```python
from build123d import *

# Parameters (mm, degrees)
BOSS_EXTRUDE1_DEPTH = 88.9
FILLET2_R           = 0.254
FILLET1_R           = 1.27
SKETCH5_W           = 7.112
SKETCH5_H           = 2.54
BOSS_EXTRUDE2_DEPTH = 177.8


with BuildPart() as part:
    # Sketch3 → Boss-Extrude1 (new body, symmetric)
    with BuildSketch(Plane.XY):
        with BuildLine():
            Line((-12.7, 12.7), (-1.796051224, 1.796051224))
            ThreePointArc((-1.796051224, 1.796051224), (-0.972015918, 2.346654013), (0, 2.54))
            Line((0, 2.54), (0, 4.826))
            Line((0, 4.826), (-1.977846327, 4.826))
            ThreePointArc((-1.977846327, 4.826), (-2.949862246, 5.019345987), (-3.773897552, 5.569948776))
            Line((-3.773897552, 5.569948776), (-7.772528286, 9.56857951))
            ThreePointArc((-7.772528286, 9.56857951), (-7.847628361, 9.946133082), (-7.527553898, 10.16))
            Line((-7.527553898, 10.16), (-3.302, 10.16))
            Line((-3.302, 10.16), (-3.302, 12.7))
            Line((-3.302, 12.7), (-12.7, 12.7))
        make_face()
    extrude(amount=BOSS_EXTRUDE1_DEPTH, both=True)

    # Fillet2
    fillet2_edges = [part.edges().sort_by_distance(p)[0] for p in [
        (-3.302, 12.7, 0),
        (-3.302, 10.16, 0),
    ]]
    fillet(fillet2_edges, radius=FILLET2_R)

    # Mirror1: part across plane


with BuildPart() as part_1:
    add(part.part)
    add(part.part.mirror(Plane(origin=(0, 0, 88.9), x_dir=(0, 0, 1), z_dir=(0.707106781, 0.707106781, 0))))

    # Fillet1
    fillet1_edges = [part_1.edges().sort_by_distance(p)[0] for p in [
        (-12.7, 12.7, 0),
    ]]
    fillet(fillet1_edges, radius=FILLET1_R)

    # Mirror2: part across plane


with BuildPart() as part_2:
    add(part_1.part)
    add(part_1.part.mirror(Plane(origin=(0, 0, 88.9), x_dir=(0, 0, 1), z_dir=(0, 1, 0))))

    # Mirror5: part across plane


with BuildPart() as part_3:
    add(part_2.part)
    add(part_2.part.mirror(Plane(origin=(0, 0, 88.9), x_dir=(0, 0, 1), z_dir=(-1, 0, 0))))

    # Sketch5 → Boss-Extrude2 (add, through all)
    with BuildSketch(Plane.XY.offset(88.9)):
        with Locations((0, -11.43)):
            Rectangle(SKETCH5_W, SKETCH5_H)
    extrude(amount=-BOSS_EXTRUDE2_DEPTH)


solid = part_3.part
```
Verification items for the finished model (mm, model axes). A direction names the side the tool comes from. Coordinates: 2 decimals unless noted, no trailing zeros. Answer in a Markdown table with one row per item.
1) Depth check by flat-ended pin: P1, Ø2, axis at x = -9.5, y = -2.5, coming from the -Z side; P2, Ø4.5, axis at y = 0, z = 18.5, coming from the -X side; P3, Ø1.2, axis at x = 0, z = -38.5, coming from the +Y side. Enter the tip coordinate at first touch or a pass-through.
The answers:
| item | result |
|---|---|
| P1 | passes through |
| P2 | stops at x = -4.84 |
| P3 | stops at y = 4.83 |
2) Access from +Z, -Z, +X, -X, +Y, -Y to the whole of each face (thin tool, end or side, straight path). Record for faces 1 (the face through (4.826, 0, 1)), 2 (the face through (-10.16, -6, 1)), 3 (the face through (0, 4.826, 1)).
The answers:
| item | result |
|---|---|
| face 1 | +Z, -Z, +X |
| face 2 | +Z, -Z |
| face 3 | +Z, -Z, +Y |
3) Section check A-A (z = 73). Give the number of separate pieces and of enclosed holes in the cut face, and give its area (3 significant figures).
The answers:
| item | result |
|---|---|
| separate pieces | 1 |
| enclosed holes | 2 |
| area | 332 mm2 |
4) Scan lines: line 1 along Y through (x, z) = (-6.5, 30); line 2 along X through (y, z) = (7, -25); line 3 along X through (y, z) = (9.75, 66). Record each from-to range of solid material in increasing order. Write a range as from..to.
The answers:
| item | result |
|---|---|
| line 1 | y = -12.7..-10.16, -8.3..-4.7, 4.7..8.3, 10.16..12.7 |
| line 2 | x = -12.7..-10.16, -8.8..-5.2, 5.2..8.8, 10.16..12.7 |
| line 3 | x = -12.7..-7.87, 7.87..12.7 |
